The model under review builds one solid part; all positions refer to its coordinate system, in mm. Coordinates: 2 decimals unless noted, no trailing zeros. Write each loop counter-clockwise with the first axis right and the second up, starting at its lowest first coordinate (ties: lowest second). Pieces come first, ordered by that corner, then holes. Notation, with made-up numbers: M 24,61 L 64,61 A21 cw 64,94 Z; hole C -6.5,25 d1. An arc over 180 degrees is marked long. Answer as a JSON object with one key per item and string values.
```python
from build123d import *

# Parameters (mm, degrees)
F1_DEPTH = 7


with BuildPart() as f1:
    # F0 (on Top) → F1 (new body)
    with BuildSketch(Plane.XY):
        with BuildLine():
            ThreePointArc((0, 11.125), (7.8665629407, 7.8665629407), (11.125, 0))
            ThreePointArc((11.125, 0), (7.8665629407, -7.8665629407), (0, -11.125))
            Line((0, -11.125), (0, -14.935))
            add(Edge.make_bspline(
                [(0.2975305523, -14.7281560773), (0.1976224081, -14.7964212888), (0.098439929, -14.8653652618), (0, -14.935)],
                knots=[0.9970613329, 0.9970613329, 0.9970613329, 0.9970613329, 1, 1, 1, 1], degree=3))
            add(Edge.make_bspline(
                [(0.2975305523, -14.7281560773), (7.3951181082, -9.7951650898), (11.9191993362, -6.7662998847), (17.3106230519, -8.3854462868)],
                knots=[0.003112202, 0.003112202, 0.003112202, 0.003112202, 0.226966528, 0.226966528, 0.226966528, 0.226966528], degree=3))
            add(Edge.make_bspline(
                [(36.9228658424, -1.1001812607), (33.3191993332, -4.9864728132), (25.4350438971, -6.457479873), (17.3106230519, -8.3854462868)],
                knots=[0.6774767782, 0.6774767782, 0.6774767782, 0.6774767782, 0.8599164447, 0.8599164447, 0.8599164447, 0.8599164447], degree=3))
            ThreePointArc((36.9228658424, -1.1001812607), (36.9392531167, 0), (36.9228658424, 1.1001812607))
            add(Edge.make_bspline(
                [(36.9228658424, 1.1001812607), (33.3191993332, 4.9864728132), (25.4350438971, 6.457479873), (17.3106230519, 8.3854462868)],
                knots=[0.6774767782, 0.6774767782, 0.6774767782, 0.6774767782, 0.8599164447, 0.8599164447, 0.8599164447, 0.8599164447], degree=3))
            add(Edge.make_bspline(
                [(0.2975305523, 14.7281560773), (7.3951181082, 9.7951650898), (11.9191993362, 6.7662998847), (17.3106230519, 8.3854462868)],
                knots=[0.003112202, 0.003112202, 0.003112202, 0.003112202, 0.226966528, 0.226966528, 0.226966528, 0.226966528], degree=3))
            add(Edge.make_bspline(
                [(0.2975305523, 14.7281560773), (0.1976224081, 14.7964212888), (0.098439929, 14.8653652618), (0, 14.935)],
                knots=[0.9970613329, 0.9970613329, 0.9970613329, 0.9970613329, 1, 1, 1, 1], degree=3))
            Line((0, 14.935), (0, 11.125))
        make_face()
        with BuildLine():
            ThreePointArc((0, -11.125), (-11.125, 0), (0, 11.125))
            Line((0, 11.125), (0, 14.935))
            add(Edge.make_bspline(
                [(-0.2975305523, 14.7281560773), (-0.1976224081, 14.7964212888), (-0.098439929, 14.8653652618), (0, 14.935)],
                knots=[0.9970613329, 0.9970613329, 0.9970613329, 0.9970613329, 1, 1, 1, 1], degree=3))
            add(Edge.make_bspline(
                [(-0.2975305523, 14.7281560773), (-7.3951181082, 9.7951650898), (-11.9191993362, 6.7662998847), (-17.3106230519, 8.3854462868)],
                knots=[0.003112202, 0.003112202, 0.003112202, 0.003112202, 0.226966528, 0.226966528, 0.226966528, 0.226966528], degree=3))
            add(Edge.make_bspline(
                [(-36.9228658424, 1.1001812607), (-33.3191993332, 4.9864728132), (-25.4350438971, 6.457479873), (-17.3106230519, 8.3854462868)],
                knots=[0.6774767782, 0.6774767782, 0.6774767782, 0.6774767782, 0.8599164447, 0.8599164447, 0.8599164447, 0.8599164447], degree=3))
            ThreePointArc((-36.9228658424, 1.1001812607), (-36.9392531167, 0), (-36.9228658424, -1.1001812607))
            add(Edge.make_bspline(
                [(-36.9228658424, -1.1001812607), (-33.3191993332, -4.9864728132), (-25.4350438971, -6.457479873), (-17.3106230519, -8.3854462868)],
                knots=[0.6774767782, 0.6774767782, 0.6774767782, 0.6774767782, 0.8599164447, 0.8599164447, 0.8599164447, 0.8599164447], degree=3))
            add(Edge.make_bspline(
                [(-0.2975305523, -14.7281560773), (-7.3951181082, -9.7951650898), (-11.9191993362, -6.7662998847), (-17.3106230519, -8.3854462868)],
                knots=[0.003112202, 0.003112202, 0.003112202, 0.003112202, 0.226966528, 0.226966528, 0.226966528, 0.226966528], degree=3))
            add(Edge.make_bspline(
                [(-0.2975305523, -14.7281560773), (-0.1976224081, -14.7964212888), (-0.098439929, -14.8653652618), (0, -14.935)],
                knots=[0.9970613329, 0.9970613329, 0.9970613329, 0.9970613329, 1, 1, 1, 1], degree=3))
            Line((0, -14.935), (0, -11.125))
        make_face()
        with BuildLine():
            add(Edge.make_bspline(
                [(0, -14.935), (-0.0996804425, -14.865688897), (-0.1988542112, -14.796738465), (-0.2975305523, -14.7281560773)],
                knots=[0, 0, 0, 0, 0.003112202, 0.003112202, 0.003112202, 0.003112202], degree=3))
            add(Edge.make_bspline(
                [(-0.2975305523, -14.7281560773), (-0.1976224081, -14.7964212888), (-0.098439929, -14.8653652618), (0, -14.935)],
                knots=[0.9970613329, 0.9970613329, 0.9970613329, 0.9970613329, 1, 1, 1, 1], degree=3))
        make_face()
        with BuildLine():
            add(Edge.make_bspline(
                [(-36.9228658424, 1.1001812607), (-33.3191993332, 4.9864728132), (-25.4350438971, 6.457479873), (-17.3106230519, 8.3854462868)],
                knots=[0.6774767782, 0.6774767782, 0.6774767782, 0.6774767782, 0.8599164447, 0.8599164447, 0.8599164447, 0.8599164447], degree=3))
            add(Edge.make_bspline(
                [(-17.3106230519, 8.3854462868), (-17.3759482788, 8.4050646867), (-22.8109780057, 10.0907940795), (-29.1662144452, 16.5153198792), (-33.7854139507, 14.935)],
                knots=[0.226966528, 0.226966528, 0.226966528, 0.226966528, 0.2296788607, 0.4521923767, 0.4521923767, 0.4521923767, 0.4521923767], degree=3))
            ThreePointArc((-33.7854139507, 14.935), (-36.0245160996, 8.1696181434), (-36.9228658424, 1.1001812607))
        make_face()
        with BuildLine():
            add(Edge.make_bspline(
                [(17.3106230519, 8.3854462868), (17.3759482788, 8.4050646867), (22.8109780057, 10.0907940795), (29.1662144452, 16.5153198792), (33.7854139507, 14.935)],
                knots=[0.226966528, 0.226966528, 0.226966528, 0.226966528, 0.2296788607, 0.4521923767, 0.4521923767, 0.4521923767, 0.4521923767], degree=3))
            add(Edge.make_bspline(
                [(36.9228658424, 1.1001812607), (33.3191993332, 4.9864728132), (25.4350438971, 6.457479873), (17.3106230519, 8.3854462868)],
                knots=[0.6774767782, 0.6774767782, 0.6774767782, 0.6774767782, 0.8599164447, 0.8599164447, 0.8599164447, 0.8599164447], degree=3))
            ThreePointArc((36.9228658424, 1.1001812607), (36.0245160996, 8.1696181434), (33.7854139507, 14.935))
        make_face()
        with BuildLine():
            add(Edge.make_bspline(
                [(-17.3106230519, -8.3854462868), (-17.3759482788, -8.4050646867), (-22.8109780057, -10.0907940795), (-29.1662144452, -16.5153198792), (-33.7854139507, -14.935)],
                knots=[0.226966528, 0.226966528, 0.226966528, 0.226966528, 0.2296788607, 0.4521923767, 0.4521923767, 0.4521923767, 0.4521923767], degree=3))
            add(Edge.make_bspline(
                [(-36.9228658424, -1.1001812607), (-33.3191993332, -4.9864728132), (-25.4350438971, -6.457479873), (-17.3106230519, -8.3854462868)],
                knots=[0.6774767782, 0.6774767782, 0.6774767782, 0.6774767782, 0.8599164447, 0.8599164447, 0.8599164447, 0.8599164447], degree=3))
            ThreePointArc((-36.9228658424, -1.1001812607), (-36.0245160996, -8.1696181434), (-33.7854139507, -14.935))
        make_face()
        with BuildLine():
            add(Edge.make_bspline(
                [(36.9228658424, -1.1001812607), (33.3191993332, -4.9864728132), (25.4350438971, -6.457479873), (17.3106230519, -8.3854462868)],
                knots=[0.6774767782, 0.6774767782, 0.6774767782, 0.6774767782, 0.8599164447, 0.8599164447, 0.8599164447, 0.8599164447], degree=3))
            add(Edge.make_bspline(
                [(17.3106230519, -8.3854462868), (17.3759482788, -8.4050646867), (22.8109780057, -10.0907940795), (29.1662144452, -16.5153198792), (33.7854139507, -14.935)],
                knots=[0.226966528, 0.226966528, 0.226966528, 0.226966528, 0.2296788607, 0.4521923767, 0.4521923767, 0.4521923767, 0.4521923767], degree=3))
            ThreePointArc((33.7854139507, -14.935), (36.0245160996, -8.1696181434), (36.9228658424, -1.1001812607))
        make_face()
    extrude(amount=F1_DEPTH)


solid = f1.part
```
(1) For pin 1 Ø3 at (x, z) = (29, 4.5) entering from -Y; pin 2 Ø1.5 at (y, z) = (-5.5, 3.5) entering from +X; pin 3 Ø3 at (x, z) = (4.5, 5) entering from +Y, all flat-tipped, find the tip position at first contact; note any pin that passes through.
Results list:
{"pin 1": "y = -14.95", "pin 2": "x = 36.63", "pin 3": "y = 12.87"}
(2) Add section A-A on y = 0. Give the boundary of the cut face in (x, z) (3 decimals).
Results list:
{"outline": "M -36.939,0 L -11.125,0 L -11.125,7 L -36.939,7 Z; M 11.125,0 L 36.939,0 L 36.939,7 L 11.125,7 Z"}
(3) Draft analysis for pull direction X (two halves, no side actions). For faces 1 (the face through (-9, -7, 0)), 2 (the face through (10.86, 2.41, 3.45)), state which applies: released by +X, released by -X, zero draft, split by the parting line, or undercut.
Results list:
{"face 1": "zero draft", "face 2": "undercut"}
(4) Add section B-B on y = 6. Give the boundary of the cut face in (x, z).
Results list:
{"outline": "M -36.45,0 L -9.37,0 L -9.37,7 L -36.45,7 Z; M 9.37,0 L 36.45,0 L 36.45,7 L 9.37,7 Z"}
(5) Add section C-C on y = 12. Count the separate pieces of the cut face and the enclosed holes in it, and give its area (3 significant figures).
Results list:
{"separate pieces": "3", "enclosed holes": "0", "area": "208 mm²"}
(6) Wall thickness on line 1 along X through (y, z) = (0, 2.75) (3 decimals); line 2 along X through (y, z) = (10, 1.25) (3 decimals); line 3 along X through (y, z) = (12.5, 5.5): over which ranges is each line inside the solid? List them lowest first. Write a range as from..to.
Results list:
{"line 1": "-36.939..-11.125, 11.125..36.939", "line 2": "-35.56..-20.943, -7.61..-4.875, 4.875..7.61, 20.943..35.56", "line 3": "-34.76..-25.19, -3.55..3.55, 25.19..34.76"}
